Solid Edge part; units mm, degrees
sketch "Sketch1" plane through (0, 0, 0) normal (0, -1, 0) x (1, 0, 0)
  arc A0 (0, 10) -> (5, -8.6603) centre (0, 0) cw
  line L0 (5, -8.6603) -> (4, -8.6603)
  line L1 (4, -8.6603) -> (4, -28.6603)
  line L2 (4, -28.6603) -> (0, -28.6603)
  dimension "D1" = 5
  dimension "D2" = 4
  dimension "D3" = 4
revolve "RevolvedProtrusion1" add sketch "Sketch1" angle 360 about axis through (0, 0, 10) along (0, 0, -1)
sketch "Sketch2" plane through (0, 0, 0) normal (1, 0, 0) x (0, 1, 0)
  line L0 (5, -8.6603) -> (11.9647, -8.6603)
  line L1 (11.9647, -8.6603) -> (11.9647, 12.055)
  line L2 (11.9647, 12.055) -> (5, 12.055)
  line L3 (5, 12.055) -> (5, -8.6603)
  line L4 (-5, -8.6603) -> (-11.8811, -8.6603)
  line L5 (-11.8811, -8.6603) -> (-11.8811, 12.3755)
  line L6 (-11.8811, 12.3755) -> (-5, 12.3755)
  line L7 (-5, 12.3755) -> (-5, -8.6603)
extrude "Cutout1" cut sketch "Sketch2" along normal mid plane 26.6508
sketch "Sketch3" plane through (0, 0, 0) normal (0, -1, 0) x (1, 0, 0)
  arc A0 (0, 7.5) -> (0, -7.5) centre (0, 0) cw
revolve "RevolvedCutout1" cut sketch "Sketch3" angle 360 about axis through (0, 0, 6) along (0, 0, -1)
cosmetic_thread "Thread1"
properties material "Steel"
Source: CAD feature listing. Evaluate the final solid. Frame: model axes, mm. A direction names the side the tool comes from. Give positions to 0.01 mm unless a question says otherwise; leave off trailing zeros. Write each loop counter-clockwise with the first axis right and the second up, starting at its lowest first coordinate (ties: lowest second). Pieces come first, ordered by that corner, then holes. Notation, with made-up numbers: M 34,75.5 L 62,75.5 A17 cw 62,102.5 Z; hole C 57.25,22 d4. An arc over 180 degrees is marked long. Answer as a JSON object with one key per item and string values.
Q1. Cut plane C-C, the plane z = -12.5. Return the cut outline in (x, y), then the cut area to 3 significant figures.
Geometry check:
{"outline": "C 0,0 d8", "area": "50.3 mm^2"}
Q2. Access query for faces 1 (the face through (0, 0, -28.66)), 2 (the face through (-0.867, 3.905, -18.8)). Directions: +Z, -Z, +X, -X, +Y, -Y. A direction counts if a zero-diameter tool reaches every point of the face in a straight line with its end or side. Return the directions, or none.
Geometry check:
{"face 1": "-Z, +X, -X, +Y, -Y", "face 2": "-Z"}
Q3. Ray query, line 1 along X through (y, z) = (-3.25, -1.5); line 2 along Y through (x, z) = (6.25, -5.5); line 3 along Z through (x, y) = (-4.75, -1.75). Return the intervals inside material, ascending.
Geometry check:
{"line 1": "x = -9.34 to -6.59, 6.59 to 9.34", "line 2": "y = -5 to 5", "line 3": "z = -8.62 to -5.53, 5.53 to 8.62"}
Q4. Contact query for flat-ended pins moving along their axis: P1, Ø2, axis at x = -2, z = -21.5, coming from the -Y side; P2, Ø1, axis at y = 4, z = -21.5, coming from the +X side; P3, Ø8, axis at x = -4.5, z = -10, coming from the -Y side. Output: stop coordinate, or through.
Geometry check:
{"P1": "stops at y = -3.87", "P2": "stops at x = 1.94", "P3": "stops at y = -5"}
Q5. Cut plane B-B, the plane z = -2. Return the cut outline in (x, y), then the cut area to 3 significant figures.
Geometry check:
{"outline": "M -8.43,-5 L -5.22,-5 A7.23 cw -5.22,5 L -8.43,5 A9.8 ccw Z; M 5.22,-5 L 8.43,-5 A9.8 ccw 8.43,5 L 5.22,5 A7.23 cw Z", "area": "55.1 mm^2"}
